from build123d import *

# Parameters (mm, degrees)
SKETCH1_W           = 69.088
SKETCH1_H           = 27.051
BOSS_EXTRUDE1_DEPTH = 1.6
SKETCH2_W           = 4.978970029
SKETCH2_H           = 6
SKETCH2_W_2         = 3.862002759
SKETCH2_H_2         = 5.859121758
BOSS_EXTRUDE2_DEPTH = 5
SKETCH3_W           = 6.5
SKETCH3_H           = 2.717485229
BOSS_EXTRUDE3_DEPTH = 2
SKETCH4_W           = 7.179475327
SKETCH4_H           = 9.5
BOSS_EXTRUDE4_DEPTH = 2.8
SKETCH5_R           = 1
CUT_EXTRUDE1_DEPTH  = 2.6
SKETCH6_R           = 1.689834655
BOSS_EXTRUDE5_DEPTH = 4
SKETCH7_R           = 0.917545462
BOSS_EXTRUDE6_DEPTH = 4.5
SKETCH8_R           = 2.5
BOSS_EXTRUDE7_DEPTH = 2


with BuildPart() as part:
    # Sketch1 → Boss-Extrude1 (new body)
    with BuildSketch(Plane(origin=(0, 0, 0), x_dir=(1, 0, 0), z_dir=(0, 1, 0))):
        with Locations((34.544, -13.5255)):
            Rectangle(SKETCH1_W, SKETCH1_H)
    extrude(amount=BOSS_EXTRUDE1_DEPTH)

    # Sketch2 → Boss-Extrude2 (add)
    with BuildSketch(Plane(origin=(0, 0, 0), x_dir=(-1, 0, 0), z_dir=(0, -1, 0))):
        with Locations((-2.289485014, -23.251)):
            Rectangle(SKETCH2_W, SKETCH2_H)
        with Locations((-2.289485014, -3.8)):
            Rectangle(SKETCH2_W, SKETCH2_H)
        with Locations((-1.126576215, -14.111503754)):
            Rectangle(SKETCH2_W_2, SKETCH2_H_2)
    extrude(amount=BOSS_EXTRUDE2_DEPTH)

    # Sketch3 → Boss-Extrude3 (add)
    with BuildSketch(Plane(origin=(0, 0, 0), x_dir=(-1, 0, 0), z_dir=(0, -1, 0))):
        with Locations((-60.838, -0.770217549)):
            Rectangle(SKETCH3_W, SKETCH3_H)
    extrude(amount=BOSS_EXTRUDE3_DEPTH)

    # Sketch4 → Boss-Extrude4 (add)
    with BuildSketch(Plane(origin=(0, 0, 0), x_dir=(-1, 0, 0), z_dir=(0, -1, 0))):
        with Locations((-65.798262337, -21.201)):
            Rectangle(SKETCH4_W, SKETCH4_H)
    extrude(amount=BOSS_EXTRUDE4_DEPTH)

    # Sketch5 → Cut-Extrude1 (cut, through all)
    with BuildSketch(Plane(origin=(0, 0, 0), x_dir=(-1, 0, 0), z_dir=(0, -1, 0))):
        with Locations((-59.563, -24.257)):
            Circle(SKETCH5_R)
        with Locations((-50.927, -3.175)):
            Circle(SKETCH5_R)
        with Locations((-10.16, -13.716)):
            Circle(SKETCH5_R)
    extrude(amount=-CUT_EXTRUDE1_DEPTH, mode=Mode.SUBTRACT)

    # Sketch6 → Boss-Extrude5 (add)
    with BuildSketch(Plane(origin=(0, 0, 0), x_dir=(-1, 0, 0), z_dir=(0, -1, 0))):
        with Locations((-59.807454833, -7.251263164)):
            Circle(SKETCH6_R)
    extrude(amount=BOSS_EXTRUDE5_DEPTH)

    # Sketch7 → Boss-Extrude6 (add)
    with BuildSketch(Plane(origin=(0, 0, 0), x_dir=(-1, 0, 0), z_dir=(0, -1, 0))):
        with Locations((-59.438742184, -16.920616946)):
            Circle(SKETCH7_R)
    extrude(amount=BOSS_EXTRUDE6_DEPTH)

    # Sketch8 → Boss-Extrude7 (add)
    with BuildSketch(Plane.ZY.offset(0.2)):
        with Locations((3.8, -2.5)):
            Circle(SKETCH8_R)
        with Locations((23.251, -2.5)):
            Circle(SKETCH8_R)
    extrude(amount=BOSS_EXTRUDE7_DEPTH)


solid = part.part
Here's how the part is built. I have some questions about the finished solid (model axes, mm). A direction names the side the tool comes from. Give positions to 0.01 mm unless a question says otherwise; leave off trailing zeros. Order: outer loops, then holes, each group sorted by start corner. A loop starts at its lowest first (then second) coordinate and runs counter-clockwise, first axis right, second up. Notation, with made-up numbers: M -17,78 L -11,78 A23 cw -11,112 Z; hole C 3.25,-4 d9. An arc over 180 degrees is marked long. Answer as a JSON object with one key per item and string values. Group by question number.
1) On a 3-axis mill with a long thin cutter (end or side, diameter ignored), from which of +Z, -Z, +X, -X, +Y, -Y can I reach the whole of each face in a straight line? I mean faces 1 (the flat face through (-0.2, -2.3, 6.5)), 2 (the flat face through (2, -2, 6.8)), 3 (the flat face through (64.088, -1, 1)), 4 (the flat face through (66, -1, 25.951)). Say none if no direction works.
2) Please list where these lines run through material, in increasing order: L1, parallel to X at y = -0.75, z = 17; L2, parallel to X at y = -0.5, z = 20.5; L3, parallel to Z at x = 10.16, y = 0.6. Write a range as [from, to].
3) Suppose I cut it at D-D, the plane z = 8.25. Write out the boundary of the cut face in (x, y).
4) We'd pull the mould along Z, two halves only. Please class faces 5 (the flat face through (2, -2, 20.251)), 6 (the flat face through (34, 1, 0)), 7 (the flat face through (4.779, -2, 23)): pulls with the +Z half, pulls with the -Z half, needs draft (parallel to the pull), parting line crosses it, or undercut.
5) I'm going to push flat-ended pins straight in: pin 1 Ø2 at (y, z) = (-4, 16.5) entering from +X; pin 2 Ø0.5 at (y, z) = (1, 18) entering from +X; pin 3 Ø1 at (y, z) = (-1, 1) entering from +X. Where does each tip first touch, or does it pass through?
6) Suppose I cut it at C-C, the plane x = 23.5. Write out the boundary of the cut face in (y, z), plus the area to 3 significant figures.
7) Suppose I cut it at B-B, the plane z = 19. Write out the boundary of the cut face in (x, y), plus the area to 3 significant figures.
8) Suppose I cut it at A-A, the plane x = 10.16. Write out the boundary of the cut face in (y, z), plus the area to 3 significant figures.
Results found:
{
 "1": {"face 1": "-X", "face 2": "-X, -Y", "face 3": "-Z, +X, -Y", "face 4": "+Z, +X, -Y"},
 "2": {"L1": "[-0.8, 3.06], [58.52, 60.35], [62.21, 69.39]", "L2": "[-0.2, 4.78], [62.21, 69.39]", "L3": "[0, 12.72], [14.72, 27.05]"},
 "3": {"outline": "M 0,0 L 58.44,0 L 58.44,-4 L 61.17,-4 L 61.17,0 L 69.09,0 L 69.09,1.6 L 0,1.6 Z"},
 "4": {"face 5": "undercut", "face 6": "pulls with the -Z half", "face 7": "needs draft"},
 "5": {"pin 1": "x = 60.36", "pin 2": "x = 69.09", "pin 3": "x = 64.09"},
 "6": {"outline": "M 0,0 L 1.6,0 L 1.6,27.05 L 0,27.05 Z", "area": "43.3 mm²"},
 "7": {"outline": "M 0,0 L 62.21,0 L 62.21,-2.8 L 69.39,-2.8 L 69.39,0 L 69.09,0 L 69.09,1.6 L 0,1.6 Z", "area": "131 mm²"},
 "8": {"outline": "M 0,0 L 1.6,0 L 1.6,12.72 L 0,12.72 Z; M 0,14.72 L 1.6,14.72 L 1.6,27.05 L 0,27.05 Z", "area": "40.1 mm²"}
}
